from build123d import *

# Parameters (mm, degrees)
F0_R     = 1.67
F1_DEPTH = 1.58
F2_R     = 3
F3_R     = 0.5


with BuildPart() as f1:
    # F0 (on Front) → F1 (new body)
    with BuildSketch(Plane.XZ):
        with BuildLine():
            Line((9.95, 0), (-9.95, 0))
            Line((-9.95, 0), (-9.95, -5))
            Line((-9.95, -5), (-7.05, -7.870274))
            Line((-7.05, -7.870274), (-7.05, -13.570274))
            Line((-7.05, -13.570274), (-9.805, -16.58))
            Line((-9.805, -16.58), (-9.805, -51.98))
            Line((-9.805, -51.98), (-6.57, -57.3))
            Line((-6.57, -57.3), (-3.335, -51.98))
            Line((-3.335, -51.98), (-3.335, -19.915))
            ThreePointArc((-3.335, -19.915), (0, -16.58), (3.335, -19.915))
            Line((3.335, -19.915), (3.335, -51.98))
            Line((3.335, -51.98), (6.57, -57.3))
            Line((6.57, -57.3), (9.805, -51.98))
            Line((9.805, -51.98), (9.805, -16.58))
            Line((9.805, -16.58), (7.05, -13.570274))
            Line((7.05, -13.570274), (7.05, -7.870274))
            Line((7.05, -7.870274), (9.95, -5))
            Line((9.95, -5), (9.95, 0))
        make_face()
        with Locations((-7.29, -2.11)):
            Circle(F0_R, mode=Mode.SUBTRACT)
        with Locations((7.29, -2.11)):
            Circle(F0_R, mode=Mode.SUBTRACT)
    extrude(amount=F1_DEPTH)

    # F2
    f2_edges = [f1.edges().sort_by_distance(p)[0] for p in [
        (-7.05, -0.79, -7.870274),
        (-7.05, -0.79, -13.570274),
        (7.05, -0.79, -7.870274),
        (7.05, -0.79, -13.570274),
    ]]
    fillet(f2_edges, radius=F2_R)

    # F3
    f3_edges = [f1.edges().sort_by_distance(p)[0] for p in [
        (-6.57, -0.79, -57.3),
        (6.57, -0.79, -57.3),
    ]]
    fillet(f3_edges, radius=F3_R)


solid = f1.part
Read the model definition and answer for the solid it produces. Units are mm, in the model's axes. A direction names the side the tool comes from. Give positions to 0.01 mm unless a question says otherwise; leave off trailing zeros. Write each loop counter-clockwise with the first axis right and the second up, starting at its lowest first coordinate (ties: lowest second). Pieces come first, ordered by that corner, then holes. Notation, with made-up numbers: (32, -14.75) - (79, -14.75) arc R25 cw to (79, 9.25) - close; hole circle Ø6 at (82.5, 69.25). An arc over 180 degrees is marked (long way). Answer in a Markdown table with one row per item. Add a question column.
Item 1: Find the intervals of material crossed by L1, parallel to X at y = -0.8, z = -46 (3 decimals); L2, parallel to Z at x = 7.29, y = -0.55; L3, parallel to Z at x = -7.5, y = -1, in increasing order.
Item 2: Section B-B, the plane z = -49 is taken. Write down the section's boundary in (x, y) (3 decimals), and give its area (3 significant figures).
Item 3: Flat-ended cylindrical pins translate along their axes: P1, Ø0.8, axis at y = -0.5, z = -42, coming from the +X side (3 decimals); P2, Ø0.8, axis at y = -1, z = -10.5, coming from the +X side; P3, Ø0.8, axis at y = -1, z = -10, coming from the -X side. Find the tip coordinate at first contact, or state that the pin passes through.
Item 4: Section C-C, the plane y = -0.75 is taken. Write down the section's boundary in (x, z) (3 decimals), and give its area (3 significant figures).
Item 5: A tool of negligible diameter and unlimited length cuts with its end or side. For faces 1 (the face through (7.05, -1, -11)), 2 (the face through (-8.96, -0.78, -5.98)), 3 (the face through (4.72, -0.78, -54.26)), 4 (the face through (-9.805, -1, -34)), from which of +Z, -Z, +X, -X, +Y, -Y can it reach the whole face along a straight path? Write none if from no direction.
Item 6: Section A-A, the plane z = -2.11 is taken. Write down the section's boundary in (x, y).
Item 7: Section D-D, the plane x = 0 is taken. Write down the section's boundary in (y, z), and give its area (3 significant figures).
Item 8: Determine the mould class of faces 5 (the face through (-0.07, -0.78, -16.58)), 6 (the face through (-7.29, -0.8, -7.95)), 7 (the face through (0, -1, 0)), 8 (the face through (8.835, -0.779, -15.52)) for opening direction Z: pulls with the +Z half, pulls with the -Z half, needs draft (parallel to the pull), parting line crosses it, or undercut.
Recorded:
| question | item | result |
|---|---|---|
| 1 | L1 | x = -9.805 to -3.335, 3.335 to 9.805 |
| 1 | L2 | z = -56.12 to -13.58, -7.95 to -3.78, -0.44 to 0 |
| 1 | L3 | z = -55.77 to -13.98, -7.54 to -3.77, -0.45 to 0 |
| 2 | outline | (-9.805, -1.58) - (-3.335, -1.58) - (-3.335, 0) - (-9.805, 0) - close; (3.335, -1.58) - (9.805, -1.58) - (9.805, 0) - (3.335, 0) - close |
| 2 | area | 20.4 mm2 |
| 3 | P1 | stops at x = 9.805 |
| 3 | P2 | stops at x = 7.05 |
| 3 | P3 | stops at x = -7.05 |
| 4 | outline | (-9.95, -5) - (-7.94, -6.99) arc R3 cw to (-7.05, -9.122) - (-7.05, -12.405) arc R3 cw to (-7.837, -14.43) - (-9.805, -16.58) - (-9.805, -51.98) - (-6.997, -56.597) arc R0.5 ccw to (-6.143, -56.597) - (-3.335, -51.98) - (-3.335, -19.915) arc R3.335 cw to (3.335, -19.915) - (3.335, -51.98) - (6.143, -56.597) arc R0.5 ccw to (6.997, -56.597) - (9.805, -51.98) - (9.805, -16.58) - (7.837, -14.43) arc R3 cw to (7.05, -12.405) - (7.05, -9.122) arc R3 cw to (7.94, -6.99) - (9.95, -5) - (9.95, 0) - (-9.95, 0) - close; hole circle Ø3.34 at (-7.29, -2.11); hole circle Ø3.34 at (7.29, -2.11) |
| 4 | area | 760 mm2 |
| 5 | face 1 | +X, +Y, -Y |
| 5 | face 2 | -X, +Y, -Y |
| 5 | face 3 | -Z, +Y, -Y |
| 5 | face 4 | -Z, -X, +Y, -Y |
| 6 | outline | (-9.95, -1.58) - (-8.96, -1.58) - (-8.96, 0) - (-9.95, 0) - close; (-5.62, -1.58) - (5.62, -1.58) - (5.62, 0) - (-5.62, 0) - close; (8.96, -1.58) - (9.95, -1.58) - (9.95, 0) - (8.96, 0) - close |
| 7 | outline | (-1.58, -16.58) - (0, -16.58) - (0, 0) - (-1.58, 0) - close |
| 7 | area | 26.2 mm2 |
| 8 | face 5 | pulls with the -Z half |
| 8 | face 6 | undercut |
| 8 | face 7 | pulls with the +Z half |
| 8 | face 8 | undercut |
